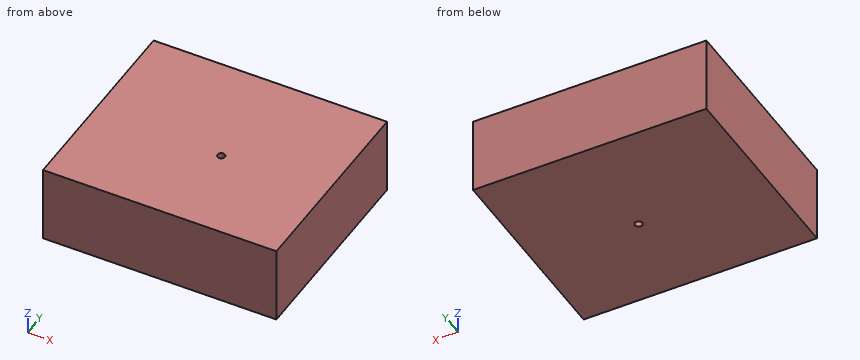
from build123d import *

# Parameters (mm, degrees)
F0_W          = 119.913816
F0_H          = 104.215179
F1_DEPTH      = 40
F2_R          = 1.858355
F3_DEPTH      = 32.004
F3_DEPTH_BACK = 58.674


with BuildPart() as f1:
    # F0 (on Top) → F1 (new body)
    with BuildSketch(Plane.XY):
        with Locations((-5.839467, 4.778015)):
            Rectangle(F0_W, F0_H)
    extrude(amount=F1_DEPTH)

    # F2 (on face) → F3 (cut, two sides)
    with BuildSketch(Plane.XY.offset(40)) as f3_sk:
        Circle(F2_R)
    extrude(amount=F3_DEPTH, mode=Mode.SUBTRACT)
    extrude(f3_sk.sketch, amount=-F3_DEPTH_BACK, mode=Mode.SUBTRACT)


solid = f1.part
CAD build for the part. Positions are in the model's coordinates, mm. Round coordinates to 2 decimals unless told otherwise and drop trailing zeros. Write each loop counter-clockwise with the first axis right and the second up, starting at its lowest first coordinate (ties: lowest second). Pieces come first, ordered by that corner, then holes.
(1) Probe line 1 along Y through (x, z) = (0, 10.5); line 2 along Y through (x, z) = (1, 32.5). List the from-to ranges inside material, lowest first.
(2) Slice it at A-A, the plane x = 0. Write the cut outline in (y, z).
(3) Slice it at B-B, the plane y = 0. Write the cut outline in (x, z), and give its area (3 significant figures).
From the geometry:
1. line 1: y = -47.33 to -1.86, 1.86 to 56.89
1. line 2: y = -47.33 to -1.57, 1.57 to 56.89
2. outline: (-47.33, 0) - (-1.86, 0) - (-1.86, 40) - (-47.33, 40) - close; (1.86, 0) - (56.89, 0) - (56.89, 40) - (1.86, 40) - close
3. outline: (-65.8, 0) - (-1.86, 0) - (-1.86, 40) - (-65.8, 40) - close; (1.86, 0) - (54.12, 0) - (54.12, 40) - (1.86, 40) - close
3. area: 4,650 mm2
